Verification items for the finished model (mm, model axes). A direction names the side the tool comes from. Coordinates: 2 decimals unless noted, no trailing zeros. Loops run counter-clockwise (first coordinate to the right, second up) from the corner with the lowest first, then second, coordinate; pieces in that order, holes last. Notation, with made-up numbers: (-36.5, 32) - (18.5, 32) arc R19 cw to (18.5, 66) - close; hole circle Ø4 at (64.5, -39). An arc over 180 degrees is marked (long way). Answer as CSV lines item,"result". Start each with the question number.
1. Cross-section at A-A (x = -4.5). Enter the section's corners in (y, z), plus the area to 3 significant figures.
2. Set-up check for faces 4 (the flat face through (-3, 13.5, 125)), 5 (the flat face through (-4, -12.5, 125)), 6 (the flat face through (-7.5, -15, 125)): record each of +Z, -Z, +X, -X, +Y, -Y from which the full face is reachable in a straight line by a thin tool's end or side.
3. Gauge pin test, flat ends, axial feed: P1, Ø1, axis at x = -5, y = -11.5, coming from the -Z side; P2, Ø1, axis at y = 16.5, z = 151, coming from the +X side; P3, Ø0.5, axis at x = -0.5, z = 137, coming from the -Y side; P4, Ø4.5, axis at x = -2.5, z = 118, coming from the +Y side. Record the tip position at first contact, or that the pin passes through.
4. Cross-section at C-C (z = 126). Enter the section's corners in (x, y).
5. Release check for a two-part mould opening along Y. For faces 1 (the flat face through (-3, -13.5, 125)), 2 (the flat face through (-0.7, -1.2, 0)), 3 (the flat face through (-1, 0, 125)) record: pulls with the +Y half, pulls with the -Y half, needs draft (parallel to the pull), parting line crosses it, or undercut.
6. Cross-section at B-B (z = 214.5). Enter the section's corners in (x, y), plus the area to 3 significant figures.
7. Material ranges on line 1 (Y direction, x = -3.25, z = 238.5); line 2 (Y direction, x = -7, z = 242.5); line 3 (X direction, y = -11, z = 47), recorded low to high. Write a range as [from, to].
```python
from build123d import *

# Parameters (mm, degrees)
EXTRUDE_THIN1_DEPTH = 449.2625
CUT_EXTRUDE1_START  = -8.5
CUT_EXTRUDE1_DEPTH  = 9.5
LPATTERN1_COUNT     = 18
LPATTERN1_PITCH     = 25
FILLET1_R           = 0.5
SKETCH5_W           = 13.158199176
SKETCH5_H           = 40.042206119
CUT_EXTRUDE2_DEPTH  = 195.2625


with BuildPart() as part:
    # Sketch3 → Extrude-Thin1 (new body)
    with BuildSketch(Plane.XY):
        Polygon((-6.5, 17.5), (-6.5, 13.5), (0, 13.5), (0, -13.5), (-6.5, -13.5), (-6.5, -17.5), (-7.5, -17.5), (-7.5, -12.5), (-1, -12.5), (-1, 12.5), (-7.5, 12.5), (-7.5, 17.5), align=None)
    extrude(amount=EXTRUDE_THIN1_DEPTH)

    # Sketch4 → Cut-Extrude1 (cut)
    with BuildSketch(Plane(origin=(0, 0, 0), x_dir=(0, 0, -1), z_dir=(1, 0, 0)).offset(CUT_EXTRUDE1_START)):
        with BuildLine():
            Line((-6.65, -3.15), (-18.35, -3.15))
            ThreePointArc((-18.35, -3.15), (-21.5, 0), (-18.35, 3.15))
            Line((-18.35, 3.15), (-6.65, 3.15))
            ThreePointArc((-6.65, 3.15), (-3.5, 0), (-6.65, -3.15))
        make_face()
    cut_extrude1 = extrude(amount=CUT_EXTRUDE1_DEPTH, mode=Mode.SUBTRACT)

    # LPattern1: Cut-Extrude1 ×18
    with Locations(*[(0, 0, i * LPATTERN1_PITCH) for i in range(1, LPATTERN1_COUNT)]):
        add(cut_extrude1, mode=Mode.SUBTRACT)

    # Fillet1
    fillet1_edges = [part.edges().sort_by_distance(p)[0] for p in [
        (-6.5, 13.5, 224.63125),
        (0, 13.5, 224.63125),
        (0, -13.5, 224.63125),
        (-6.5, -13.5, 224.63125),
        (-7.5, -12.5, 224.63125),
        (-1, -12.5, 224.63125),
        (-1, 12.5, 224.63125),
        (-7.5, 12.5, 224.63125),
    ]]
    fillet(fillet1_edges, radius=FILLET1_R)

    # Sketch5 → Cut-Extrude2 (cut)
    with BuildSketch(Plane.XY.offset(449.2625)):
        with Locations((-4.513311055, 1.584769395)):
            Rectangle(SKETCH5_W, SKETCH5_H)
    extrude(amount=-CUT_EXTRUDE2_DEPTH, mode=Mode.SUBTRACT)


solid = part.part
```
Values follow:
1,outline,"(-13.5, 0) - (-12.5, 0) - (-12.5, 254) - (-13.5, 254) - close; (12.5, 0) - (13.5, 0) - (13.5, 254) - (12.5, 254) - close"
1,area,"508 mm²"
2,face 4,"+Z, -Z, +X, +Y"
2,face 5,"+Z, -Z, -X"
2,face 6,"+Z, -Z, -X, +Y, -Y"
3,P1,"passes through"
3,P2,"stops at x = -6.5"
3,P3,"stops at y = -13.5"
3,P4,"stops at y = 13.5"
4,outline,"(-7.5, -17.5) - (-6.5, -17.5) - (-6.5, -14) arc R0.5 cw to (-6, -13.5) - (-0.5, -13.5) arc R0.5 ccw to (0, -13) - (0, 13) arc R0.5 ccw to (-0.5, 13.5) - (-6, 13.5) arc R0.5 cw to (-6.5, 14) - (-6.5, 17.5) - (-7.5, 17.5) - (-7.5, 13) arc R0.5 ccw to (-7, 12.5) - (-1.5, 12.5) arc R0.5 cw to (-1, 12) - (-1, -12) arc R0.5 cw to (-1.5, -12.5) - (-7, -12.5) arc R0.5 ccw to (-7.5, -13) - close"
5,face 1,"pulls with the -Y half"
5,face 2,"needs draft"
5,face 3,"undercut"
6,outline,"(-7.5, -17.5) - (-6.5, -17.5) - (-6.5, -14) arc R0.5 cw to (-6, -13.5) - (-0.5, -13.5) arc R0.5 ccw to (0, -13) - (0, -3.15) - (-1, -3.15) - (-1, -12) arc R0.5 cw to (-1.5, -12.5) - (-7, -12.5) arc R0.5 ccw to (-7.5, -13) - close; (-7.5, 13) arc R0.5 ccw to (-7, 12.5) - (-1.5, 12.5) arc R0.5 cw to (-1, 12) - (-1, 3.15) - (0, 3.15) - (0, 13) arc R0.5 ccw to (-0.5, 13.5) - (-6, 13.5) arc R0.5 cw to (-6.5, 14) - (-6.5, 17.5) - (-7.5, 17.5) - close"
6,area,"41.7 mm²"
7,line 1,"y = [-13.5, -12.5], [12.5, 13.5]"
7,line 2,"y = [-17.5, -12.5], [12.5, 17.5]"
7,line 3,"x = [-1, 0]"
